Geometry: final body of the model. Coordinates: model frame, mm. A direction names the side the tool comes from. Give positions to 0.01 mm unless a question says otherwise; leave off trailing zeros. Write each loop counter-clockwise with the first axis right and the second up, starting at its lowest first coordinate (ties: lowest second). Pieces come first, ordered by that corner, then holes. Notation, with made-up numbers: (6, -5.75) -> (58, -5.75) arc R26 cw to (58, 31.25) -> close; hole circle Ø2 at (79, -22.75). An arc over 180 degrees is marked (long way). Answer as a JSON object with one key per item and string values. Group by question number.
(1) Section query B-B on z = 7.5. Output: boundary loops of the cut face in (x, y).
(2) Contact query for flat-ended pins moving along their axis: pin 1 Ø18 at (y, z) = (-385.5, -53.5) entering from -X; pin 2 Ø8 at (x, y) = (49, -178) entering from -Z; pin 3 Ø3 at (y, z) = (387, -60.5) entering from +X. Output: stop coordinate, or through.
(3) Material intervals for probe 1 along X at (y, z) = (378.5, -38); probe 2 along Z at (x, y) = (15.5, -809.5); probe 3 along X at (y, z) = (-10.5, 61), sorted ascending.
(4) Set-up query: faces 5 (the face through (32, 15, 77)), 6 (the face through (38, 15, -57)). Return all of +Z, -Z, +X, -X, +Y, -Y with unobstructed straight access to the full face (end or side cutting, diameter ignored); none if empty.
(5) Draft query along X for faces 1 (the face through (53, -1050, -6)), 2 (the face through (54, 15, 13)), 3 (the face through (39.5, 15, -57)), 4 (the face through (31, 15, 75.5)). Return one class per face: +X half, -X half, draft (parallel to the pull), parting line (faces both ways), or undercut.
from build123d import *

# Parameters (mm, degrees)
BASE_FLANGE1_DEPTH     = 1050
CUT_EXTRUDE3_START     = 835
CUT_EXTRUDE3_OUTLINE_W = 1.5
CUT_EXTRUDE3_OUTLINE_H = 23
CUT_EXTRUDE3_DEPTH     = 213


# Read off the part's stored shape, not the designer's step: Cut-Extrude3
# Sheet-metal steps are written as plain solids
with BuildPart() as part:
    # Sketch1 → Base-Flange1 (new, symmetric)
    with BuildSketch(Plane(origin=(0, 0, 0), x_dir=(1, 0, 0), z_dir=(0, 1, 0))):
        with BuildLine():
            Line((9.5, 65), (9.5, 74.7634))
            ThreePointArc((9.5, 74.7634), (10.155084973, 76.344915027), (11.7366, 77))
            Line((11.7366, 77), (37.2634, 77))
            ThreePointArc((37.2634, 77), (38.844915027, 76.344915027), (39.5, 74.7634))
            Line((39.5, 74.7634), (39.5, 49))
            Line((39.5, 49), (39.5, 38.8))
            ThreePointArc((39.5, 38.8), (41.269678139, 37.091041686), (42.915834526, 38.91928357))
            Line((42.915834526, 38.91928357), (42.378230266, 46.607382671))
            ThreePointArc((42.378230266, 46.607382671), (42.973636332, 48.288757532), (44.609382021, 49))
            Line((44.609382021, 49), (51.7634, 49))
            ThreePointArc((51.7634, 49), (53.344915027, 48.344915027), (54, 46.7634))
            Line((54, 46.7634), (54, -30))
            Line((54, -30), (54, -74.7634))
            ThreePointArc((54, -74.7634), (53.344915027, -76.344915027), (51.7634, -77))
            Line((51.7634, -77), (39.5, -77))
            Line((39.5, -77), (11.7366, -77))
            ThreePointArc((11.7366, -77), (10.155084973, -76.344915027), (9.5, -74.7634))
            Line((9.5, -74.7634), (9.5, -65))
            Line((9.5, -65), (11, -65))
            Line((11, -65), (11, -74.7634))
            ThreePointArc((11, -74.7634), (11.215745145, -75.284254855), (11.7366, -75.5))
            Line((11.7366, -75.5), (39.5, -75.5))
            Line((39.5, -75.5), (51.7634, -75.5))
            ThreePointArc((51.7634, -75.5), (52.284254855, -75.284254855), (52.5, -74.7634))
            Line((52.5, -74.7634), (52.5, -30))
            Line((52.5, -30), (52.5, 46.7634))
            ThreePointArc((52.5, 46.7634), (52.284254855, 47.284254855), (51.7634, 47.5))
            Line((51.7634, 47.5), (44.609382021, 47.5))
            ThreePointArc((44.609382021, 47.5), (44.070666884, 47.265759992), (43.874576341, 46.712017381))
            Line((43.874576341, 46.712017381), (44.412180601, 39.023918281))
            ThreePointArc((44.412180601, 39.023918281), (41.322027384, 35.591955445), (38, 38.8))
            Line((38, 38.8), (38, 49))
            Line((38, 49), (38, 74.7634))
            ThreePointArc((38, 74.7634), (37.784254855, 75.284254855), (37.2634, 75.5))
            Line((37.2634, 75.5), (11.7366, 75.5))
            ThreePointArc((11.7366, 75.5), (11.215745145, 75.284254855), (11, 74.7634))
            Line((11, 74.7634), (11, 65))
            Line((11, 65), (9.5, 65))
        make_face()
    extrude(amount=BASE_FLANGE1_DEPTH, both=True)

    # Cut-Extrude3 outline → Cut-Extrude3 (cut)
    with BuildSketch(Plane(origin=(0, 0, 0), x_dir=(1, 0, 0), z_dir=(0, 1, 0)).offset(CUT_EXTRUDE3_START)):
        with Locations((38.75, 57.5)):
            Rectangle(CUT_EXTRUDE3_OUTLINE_W, CUT_EXTRUDE3_OUTLINE_H)
        with BuildLine():
            Line((48, 47.5), (48, 49))
            Line((48, 49), (44.609382021, 49))
            ThreePointArc((44.609382021, 49), (42.973636332, 48.288757532), (42.378230266, 46.607382671))
            Line((42.378230266, 46.607382671), (42.428019372, 45.895365289))
            Line((42.428019372, 45.895365289), (43.924365447, 46))
            Line((43.924365447, 46), (43.874576341, 46.712017381))
            ThreePointArc((43.874576341, 46.712017381), (44.070666884, 47.265759992), (44.609382021, 47.5))
            Line((44.609382021, 47.5), (48, 47.5))
        make_face()
    extrude(amount=CUT_EXTRUDE3_DEPTH, mode=Mode.SUBTRACT)


solid = part.part
Answer list:
{
 "1": {"outline": "(52.5, -1050) -> (54, -1050) -> (54, 1050) -> (52.5, 1050) -> close"},
 "2": {"pin 1": "x = 38", "pin 2": "z = -49", "pin 3": "x = 39.5"},
 "3": {"probe 1": "38.1 to 39.7, 42.72 to 44.32, 52.5 to 54", "probe 2": "-77 to -75.5, 75.5 to 77", "probe 3": "52.5 to 54"},
 "4": {"face 5": "+Z, +X, -X, +Y, -Y", "face 6": "+Y, -Y"},
 "5": {"face 1": "draft", "face 2": "+X half", "face 3": "undercut", "face 4": "undercut"}
}
